from build123d import *

# Parameters (mm, degrees)
CYLINDER001_R     = 1.5
CYLINDER001_DEPTH = 10
CYLINDER_R        = 1.5
CYLINDER_DEPTH    = 10
BOX_W             = 20
BOX_H             = 15
BOX_DEPTH         = 2
PAD_DEPTH         = 14
PAD002_DEPTH      = 1.5
PAD003_DEPTH      = 1.5


with BuildPart() as cylinder001:
    # Cylinder001 → Cylinder001 (new body)
    with BuildSketch(Plane(origin=(15, 7.5, 0), x_dir=(1, 0, 0), z_dir=(0, 0, 1))):
        Circle(CYLINDER001_R)
    extrude(amount=CYLINDER001_DEPTH)


with BuildPart() as cylinder:
    # Cylinder → Cylinder (new body)
    with BuildSketch(Plane(origin=(5, 7.5, 0), x_dir=(1, 0, 0), z_dir=(0, 0, 1))):
        Circle(CYLINDER_R)
    extrude(amount=CYLINDER_DEPTH)


with BuildPart() as cut001:
    # Box → Box (new body)
    with BuildSketch(Plane.XY):
        with Locations((10, 7.5)):
            Rectangle(BOX_W, BOX_H)
    extrude(amount=BOX_DEPTH)

    # Cut: cut Cylinder
    add(cylinder.part, mode=Mode.SUBTRACT)

    # Cut001: cut Cylinder001
    add(cylinder001.part, mode=Mode.SUBTRACT)


with BuildPart() as pad:
    # Sketch → Pad (new body)
    with BuildSketch(Plane.XY):
        Polygon((0, 15), (-6.9, 15), (-6.9, 12.1), (-5.4, 12.1), (-5.4, 13.1), (-3.2, 13.1), (-3.2, 12.1), (-1.5, 12.1), (-1.5, 2.9), (-3.2, 2.9), (-3.2, 1.9), (-5.4, 1.9), (-5.4, 2.9), (-6.9, 2.9), (-6.9, 0), (0, 0), align=None)
    extrude(amount=PAD_DEPTH)


with BuildPart() as pad002:
    # Sketch001 → Pad002 (new body)
    with BuildSketch(Plane.XZ.offset(-15)):
        Polygon((0, 14), (12, 2), (0, 2), align=None)
    extrude(amount=PAD002_DEPTH)


with BuildPart() as fusion:
    # Sketch002 → Pad003 (new body)
    with BuildSketch(Plane.XZ.offset(-1.5)):
        Polygon((0, 14), (12, 2), (0, 2), align=None)
    extrude(amount=PAD003_DEPTH)

    # Fusion: union Cut001, Pad, Pad002
    add(cut001.part)
    add(pad.part)
    add(pad002.part)


solid = fusion.part
CAD build for the part. Positions are in the model's coordinates, mm. A direction names the side the tool comes from. Coordinates: 2 decimals unless noted, no trailing zeros. Write each loop counter-clockwise with the first axis right and the second up, starting at its lowest first coordinate (ties: lowest second). Pieces come first, ordered by that corner, then holes. Notation, with made-up numbers: M 5,-26.75 L 47,-26.75 A27 ccw 47,-0.75 Z; hole C 19.25,35.25 d7. An arc over 180 degrees is marked long. Return JSON: item names as keys, results as strings.
Item 1: Drop flat-ended pins along their axis: pin 1 Ø3.5 at (y, z) = (9.5, 10) entering from +X; pin 2 Ø4.5 at (y, z) = (6.5, 5.5) entering from -X; pin 3 Ø1.1 at (x, z) = (-4, 10) entering from -Y; pin 4 Ø5 at (x, z) = (15, 5.5) entering from -Y. Give the stop position or say it passes through.
Findings below:
{"pin 1": "stops at x = 0", "pin 2": "stops at x = -1.5", "pin 3": "stops at y = 0", "pin 4": "passes through"}
Item 2: Two-plate mould, pull along X, no slides. Class faces 4 (the flat face through (-5.4, 2.4, 6.9)), 5 (the flat face through (-4, 1.9, 7)), 6 (the flat face through (0, 7, 8)), 7 (the flat face through (-6, 12.1, 7)): +X half, -X half, draft (parallel to the pull), parting line (faces both ways), or undercut.
Findings below:
{"face 4": "undercut", "face 5": "undercut", "face 6": "+X half", "face 7": "draft"}
Item 3: Slice it at C-C, the plane x = 9.5. Write the cut outline in (y, z).
Findings below:
{"outline": "M 0,0 L 15,0 L 15,4.5 L 13.5,4.5 L 13.5,2 L 1.5,2 L 1.5,4.5 L 0,4.5 Z"}
Item 4: Slice it at D-D, the plane y = 3.25. Write the cut outline in (x, z), and give its area (3 significant figures).
Findings below:
{"outline": "M -1.5,0 L 20,0 L 20,2 L 0,2 L 0,14 L -1.5,14 Z", "area": "61.0 mm2"}
Item 5: Slice it at A-A, the plane x = 5. Write the cut outline in (y, z), and give its area (3 significant figures).
Findings below:
{"outline": "M 0,0 L 6,0 L 6,2 L 1.5,2 L 1.5,9 L 0,9 Z; M 9,0 L 15,0 L 15,9 L 13.5,9 L 13.5,2 L 9,2 Z", "area": "45.0 mm2"}
Item 6: Slice it at B-B, the plane z = 1. Write the cut outline in (x, y).
Findings below:
{"outline": "M -6.9,0 L 20,0 L 20,15 L -6.9,15 L -6.9,12.1 L -5.4,12.1 L -5.4,13.1 L -3.2,13.1 L -3.2,12.1 L -1.5,12.1 L -1.5,2.9 L -3.2,2.9 L -3.2,1.9 L -5.4,1.9 L -5.4,2.9 L -6.9,2.9 Z; hole C 5,7.5 d3; hole C 15,7.5 d3"}
Item 7: Probe line 1 (X direction, y = 7.5, z = 1.2); line 2 (Y direction, x = 15, z = 0.5); line 3 (Y direction, x = -2.75, z = 7.5). List the from-to ranges inside material, lowest first. Write a range as from..to.
Findings below:
{"line 1": "x = -1.5..3.5, 6.5..13.5, 16.5..20", "line 2": "y = 0..6, 9..15", "line 3": "y = 0..2.9, 12.1..15"}
Item 8: Which spindle directions (+Z, -Z, +X, -X, +Y, -Y) get a long thin tool onto all of the face, cutting with end or side? Do faces 1 (the flat face through (-1.5, 8, 7)), 2 (the flat face through (-5.4, 12.6, 6.9)), 3 (the flat face through (3, 13.5, 5)). Say none if no direction does.
Findings below:
{"face 1": "+Z, -Z, -X", "face 2": "+Z, -Z", "face 3": "+Z, +X"}
